Verification items for this drawing (mm, ordinates from the low corner). A direction names the side the tool comes from. Give positions to 0.01 mm unless a question says otherwise; leave off trailing zeros. Order: outer loops, then holes, each group sorted by start corner. A loop starts at its lowest first (then second) coordinate and runs counter-clockwise, first axis right, second up. Notation, with made-up numbers: (27, -11.5) -> (42, -11.5) arc R30 ccw to (42, 20.5) -> close; hole circle Ø9 at (-1, 66). An arc over 180 degrees is marked (long way). One line per question, with ' | ' between items.
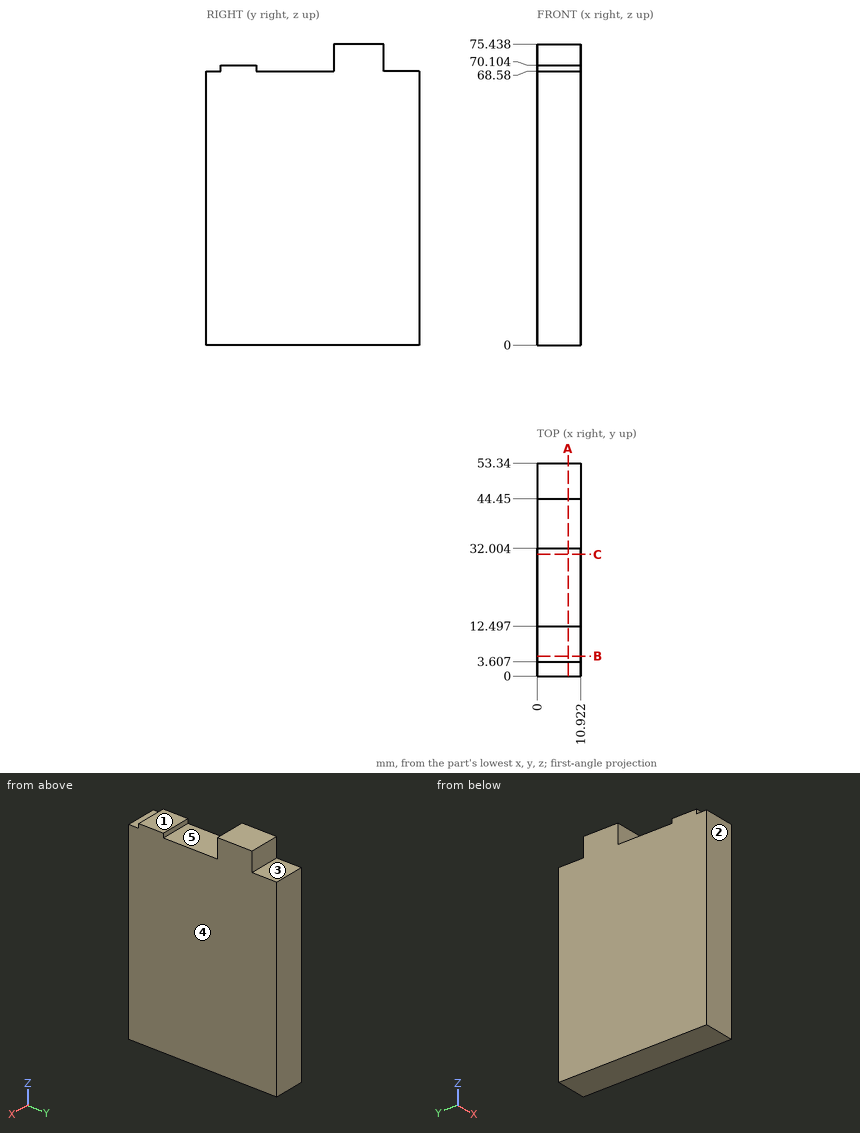
Q1. Section check A-A (x = 7.75). Enter the section's corners in (y, z).
Result sheet:
outline: (0, 0) -> (53.34, 0) -> (53.34, 68.58) -> (44.45, 68.58) -> (44.45, 75.44) -> (32, 75.44) -> (32, 68.58) -> (12.5, 68.58) -> (12.5, 70.1) -> (3.61, 70.1) -> (3.61, 68.58) -> (0, 68.58) -> close
Q2. Depth check by flat-ended pin: pin 1 Ø1.7 at (x, z) = (5, 69.5) entering from +Y; pin 2 Ø1 at (x, y) = (6, 46) entering from +Z; pin 3 Ø6 at (x, y) = (4, 6) entering from -Z; pin 4 Ø2 at (x, y) = (8.5, 9) entering from +Z. Enter the tip coordinate at first touch or a pass-through.
Result sheet:
pin 1: stops at y = 44.45 | pin 2: stops at z = 68.58 | pin 3: stops at z = 0 | pin 4: stops at z = 70.1
Q3. Section check C-C (y = 30.5). Enter the section's corners in (x, z).
Result sheet:
outline: (0, 0) -> (10.92, 0) -> (10.92, 68.58) -> (0, 68.58) -> close
Q4. Access from +Z, -Z, +X, -X, +Y, -Y to the whole of each face (thin tool, end or side, straight path). Record for the marked faces 1, 2, 3, 4 and 5.
Result sheet:
face 1: +Z, +X, -X, -Y | face 2: +Z, -Z, +X, -X, -Y | face 3: +Z, +X, -X, +Y | face 4: +Z, -Z, +X, +Y, -Y | face 5: +Z, +X, -X
Q5. Thickness scan on line 1 (Z direction, x = 3.25, y = 22.5); line 2 (Z direction, x = 3, y = 12). Record the ranges inside material, lowest first.
Result sheet:
line 1: z = 0 to 68.58 | line 2: z = 0 to 70.1
Q6. Section check B-B (y = 5). Enter the section's corners in (x, z).
Result sheet:
outline: (0, 0) -> (10.92, 0) -> (10.92, 70.1) -> (0, 70.1) -> close
